from build123d import *

# Parameters (mm, degrees)
F0_W     = 900
F0_H     = 260
F1_DEPTH = 30
F2_W     = 40
F2_H     = 40
F3_DEPTH = 450
F5_W     = 900
F5_H     = 260
F6_DEPTH = 25


with BuildPart() as f1:
    # F0 (on Top) → F1 (new body)
    with BuildSketch(Plane.XY):
        Rectangle(F0_W, F0_H)
    extrude(amount=-F1_DEPTH)

    # F2 (on Top) → F3 (join)
    with BuildSketch(Plane.XY):
        with Locations((430, 110)):
            Rectangle(F2_W, F2_H)
        with Locations((-430, 110)):
            Rectangle(F2_W, F2_H)
        with Locations((-430, -110)):
            Rectangle(F2_W, F2_H)
        with Locations((430, -110)):
            Rectangle(F2_W, F2_H)
    extrude(amount=-F3_DEPTH)

    # F5 (on offset) → F6 (join)
    with BuildSketch(Plane.XY.offset(-200)):
        Rectangle(F5_W, F5_H)
    extrude(amount=F6_DEPTH)


solid = f1.part
The listing builds one solid part. Answer for the finished solid, in the listing's coordinates (mm). A direction names the side the tool comes from. Coordinates: 2 decimals unless noted, no trailing zeros. Loops run counter-clockwise (first coordinate to the right, second up) from the corner with the lowest first, then second, coordinate; pieces in that order, holes last.
1) Find the intervals of material crossed by L1, parallel to X at y = 110, z = -103; L2, parallel to Z at x = 372, y = 5.5, in increasing order.
2) Find section A-A on z = -314.5. Write down the section's boundary in (x, y), then the cut area to 3 significant figures.
3) Find section C-C on x = -49. Write down the section's boundary in (y, z).
4) Find section B-B on y = -9. Write down the section's boundary in (x, z).
5) Determine the mould class of faces 1 (the face through (430, -110, -450)), 2 (the face through (450, -97, -174)), 3 (the face through (-6, 2, -30)) for opening direction X: pulls with the +X half, pulls with the -X half, needs draft (parallel to the pull), parting line crosses it, or undercut.
6) Find section D-D on y = 113.5. Write down the section's boundary in (x, z).
7) A tool of negligible diameter and unlimited length cuts with its end or side. For faces 4 (the face through (410, 110, -323)), 5 (the face through (410, 110, -101)), 6 (the face through (-430, -90, -323)), from which of +Z, -Z, +X, -X, +Y, -Y can it reach the whole face along a straight path? Write none if from no direction.
Values:
1. L1: x = -450 to -410, 410 to 450
1. L2: z = -200 to -175, -30 to 0
2. outline: (-450, -130) - (-410, -130) - (-410, -90) - (-450, -90) - close; (-450, 90) - (-410, 90) - (-410, 130) - (-450, 130) - close; (410, -130) - (450, -130) - (450, -90) - (410, -90) - close; (410, 90) - (450, 90) - (450, 130) - (410, 130) - close
2. area: 6,400 mm2
3. outline: (-130, -200) - (130, -200) - (130, -175) - (-130, -175) - close; (-130, -30) - (130, -30) - (130, 0) - (-130, 0) - close
4. outline: (-450, -200) - (450, -200) - (450, -175) - (-450, -175) - close; (-450, -30) - (450, -30) - (450, 0) - (-450, 0) - close
5. face 1: needs draft
5. face 2: pulls with the +X half
5. face 3: undercut
6. outline: (-450, -450) - (-410, -450) - (-410, -200) - (410, -200) - (410, -450) - (450, -450) - (450, 0) - (-450, 0) - close; hole (-410, -175) - (410, -175) - (410, -30) - (-410, -30) - close
7. face 4: -Z, +Y, -Y
7. face 5: +Y, -Y
7. face 6: -Z, +X, -X
